from build123d import *

# Parameters (mm, degrees)
Y_KSEKLIK_EKSTR_ZYON1_DEPTH = 12
IZIM2_W                     = 12
IZIM2_H                     = 15
Y_KSEKLIK_EKSTR_ZYON2_DEPTH = 71.25
IZIM3_W                     = 12
IZIM3_H                     = 42.5
Y_KSEKLIK_EKSTR_ZYON3_DEPTH = 13.75
IZIM4_W                     = 12
IZIM4_H                     = 42.5
Y_KSEKLIK_EKSTR_ZYON4_DEPTH = 13.75
F_23_0_23_AP_DELIK1_D       = 23
F_12_5_12_5_AP_DELIK1_D     = 12.5
F_12_5_12_5_AP_DELIK1_DEPTH = 83.25
RADYUS1_R                   = 3


with BuildPart() as part:
    # Çizim1 → Yükseklik-Ekstrüzyon1 (new body)
    with BuildSketch(Plane.XZ.offset(-37.9375)):
        with BuildLine():
            Line((-1.153440428, 15), (-42.076338309, 15))
            ThreePointArc((-42.076338309, 15), (-75.574161168, 8.385590262), (-42.47527254, 0))
            Line((-42.47527254, 0), (-1.153440428, 0))
            Line((-1.153440428, 0), (-1.153440428, 15))
        make_face()
    extrude(amount=-Y_KSEKLIK_EKSTR_ZYON1_DEPTH)

    # Çizim2 → Yükseklik-Ekstrüzyon2 (add)
    with BuildSketch(Plane.XZ.offset(-37.9375)):
        with Locations((-7.153440428, 7.5)):
            Rectangle(IZIM2_W, IZIM2_H)
    extrude(amount=Y_KSEKLIK_EKSTR_ZYON2_DEPTH)

    # Çizim3 → Yükseklik-Ekstrüzyon3 (add)
    with BuildSketch(Plane(origin=(0, 0, 0), x_dir=(-1, 0, 0), z_dir=(0, 0, -1))):
        with Locations((7.153440428, -12.0625)):
            Rectangle(IZIM3_W, IZIM3_H)
    extrude(amount=Y_KSEKLIK_EKSTR_ZYON3_DEPTH)

    # Çizim4 → Yükseklik-Ekstrüzyon4 (add)
    with BuildSketch(Plane.XY.offset(15)):
        with Locations((-7.153440428, -12.0625)):
            Rectangle(IZIM4_W, IZIM4_H)
    extrude(amount=Y_KSEKLIK_EKSTR_ZYON4_DEPTH)

    # Ø23.0 (23) Çap Delik1 (through all)
    with Locations(Plane.ZY.offset(13.153440428)):
        with Locations((7.5, -12.0625)):
            Hole(F_23_0_23_AP_DELIK1_D / 2)

    # Ø12.5 (12.5) Çap Delik1
    with Locations(Plane(origin=(0, 49.9375, 0), x_dir=(1, 0, 0), z_dir=(0, 1, 0))):
        with Locations((-58.080346996, -7.920331509)):
            Hole(F_12_5_12_5_AP_DELIK1_D / 2, depth=F_12_5_12_5_AP_DELIK1_DEPTH)

    # Radyus1
    radyus1_edges = [part.edges().sort_by_distance(p)[0] for p in [
        (-7.153440428, -33.3125, -13.75),
        (-7.153440428, 9.1875, -13.75),
        (-7.153440428, -33.3125, 28.75),
        (-7.153440428, 9.1875, 28.75),
    ]]
    fillet(radyus1_edges, radius=RADYUS1_R)


solid = part.part
Build history of the part. All positions in model axes, mm. A direction names the side the tool comes from. Give positions to 0.01 mm unless a question says otherwise; leave off trailing zeros. Write each loop counter-clockwise with the first axis right and the second up, starting at its lowest first coordinate (ties: lowest second). Pieces come first, ordered by that corner, then holes. Notation, with made-up numbers: (42, -38) - (80, -38) arc R21 ccw to (80, -25) - close; hole circle Ø10 at (24.25, 52.5). An arc over 180 degrees is marked (long way). Use one line per item in the form item = value. Start each with the question number.
1. Probe line 1 (Y direction, x = -3.75, z = 7.5); line 2 (X direction, y = -14, z = 20); line 3 (Y direction, x = -25.5, z = 4). List the from-to ranges inside material, lowest first. Write a range as [from, to].
2. Band-saw the part on A-A on y = -6. Write the cut outline in (x, z), plus the area to 3 significant figures.
3. 3-axis set-ups, long thin cutter, end or side, ignore diameter. For faces 5 (the face through (-13.153, 2, 7)), 6 (the face through (-7, 9.188, -5)), 7 (the face through (-17, 39, 15)), 8 (the face through (-7.069, -32.41, 27.895)): which of +Z, -Z, +X, -X, +Y, -Y reach the whole face in a straight line?
4. Band-saw the part on B-B on z = 17. Write the cut outline in (x, y).
5. Two-plate mould, pull along Y, no slides. Class faces 1 (the face through (-45, 37.938, 8)), 2 (the face through (-7.069, -2.366, 1.318)), 3 (the face through (-18, 39, 0)), 4 (the face through (-7, 9.188, 20)): released by +Y, released by -Y, zero draft, split by the parting line, or undercut.
6. Drop flat-ended pins along their axis: pin 1 Ø12 at (y, z) = (-6.5, 22) entering from -X; pin 2 Ø16 at (x, z) = (-58.08, 7.92) entering from -Y; pin 3 Ø3 at (x, z) = (-5, 20.5) entering from +Y. Give the stop position or say it passes through.
7. Band-saw the part on C-C on x = -58.5. Write the cut outline in (y, z), plus the area to 3 significant figures.
8. Band-saw the part on D-D on y = 41. Write the cut outline in (x, z).
Conclusion:
q1.line_1 = [-33.31, -23.56], [-0.56, 49.94]
q1.line_2 = [-13.15, -1.15]
q1.line_3 = [37.94, 49.94]
q2.outline = (-13.15, -13.75) - (-1.15, -13.75) - (-1.15, -2.27) - (-13.15, -2.27) - close; (-13.15, 17.27) - (-1.15, 17.27) - (-1.15, 28.75) - (-13.15, 28.75) - close
q2.area = 275 mm²
q3.face_5 = +Z, -Z, -X, -Y
q3.face_6 = -Z, +X, -X, +Y
q3.face_7 = +Z, +X, +Y
q3.face_8 = +Z, +X, -X, -Y
q4.outline = (-73.04, 37.94) - (-43.12, 37.94) - (-43.12, 49.94) - (-73.04, 49.94) - close; (-13.15, -33.31) - (-1.15, -33.31) - (-1.15, -18.54) - (-13.15, -18.54) - close; (-13.15, -5.58) - (-1.15, -5.58) - (-1.15, 9.19) - (-13.15, 9.19) - close
q5.face_1 = released by -Y
q5.face_2 = undercut
q5.face_3 = zero draft
q5.face_4 = released by +Y
q6.pin_1 = -13.15
q6.pin_2 = 37.94
q6.pin_3 = 9.19
q7.outline = (37.94, -9.57) - (49.94, -9.57) - (49.94, 1.68) - (37.94, 1.68) - close; (37.94, 14.16) - (49.94, 14.16) - (49.94, 25.42) - (37.94, 25.42) - close
q7.area = 270 mm²
q8.outline = (-42.48, 0) - (-1.15, 0) - (-1.15, 15) - (-42.08, 15) arc R17.5 ccw (long way) to start; hole circle Ø12.5 at (-58.08, 7.92)
